The listing builds one solid part. Answer for the finished solid, in the listing's coordinates (mm). Face numbers are marked on the shaded views. A direction names the side the tool comes from. Give positions to 0.01 mm unless a question says otherwise; leave off trailing zeros. Order: outer loops, then holes, each group sorted by start corner. A loop starts at its lowest first (then second) coordinate and runs counter-clockwise, first axis right, second up. Notation, with made-up numbers: (65, 23) - (80, 23) arc R15 ccw to (80, 52) - close; hole circle Ø3 at (-11.5, -37). An arc over 180 degrees is marked (long way). Answer in a Markdown table with one row per item. Add a question column.
```python
from build123d import *

# Parameters (mm, degrees)
BOSS_EXTRUDE1_DEPTH = 220
CUT_EXTRUDE1_REACH  = 22
SKETCH3_R           = 3
CUT_EXTRUDE2_DEPTH  = 220


with BuildPart() as part:
    # Sketch1 → Boss-Extrude1 (new body)
    with BuildSketch(Plane.XY):
        Polygon((-157.703422053, 227.136882129), (-157.703422053, 225.136882129), (-177.703422053, 225.136882129), (-177.703422053, 250.136882129), (-157.703422053, 250.136882129), (-157.703422053, 248.136882129), (-175.703422053, 248.136882129), (-175.703422053, 227.136882129), align=None)
    extrude(amount=BOSS_EXTRUDE1_DEPTH)

    # Sketch2 → Cut-Extrude1 (cut, up to next)
    with BuildSketch(Plane.ZY.offset(177.703422053), mode=Mode.PRIVATE) as cut_extrude1_sk1:
        with BuildLine():
            Line((34.406705906, 248.069619472), (185.593294094, 248.069619472))
            ThreePointArc((185.593294094, 248.069619472), (196.026031437, 237.636882129), (185.593294094, 227.204144786))
            Line((185.593294094, 227.204144786), (34.406705906, 227.204144786))
            ThreePointArc((34.406705906, 227.204144786), (25.093294094, 237.636882129), (34.406705906, 248.069619472))
        make_face()
    cut_extrude1_tool1 = extrude(cut_extrude1_sk1.sketch, amount=-CUT_EXTRUDE1_REACH, mode=Mode.PRIVATE) & part.part
    add(cut_extrude1_tool1.solids().sort_by_distance((-177.703422, 237.636882, 110.543615))[0], mode=Mode.SUBTRACT)

    # Sketch3 → Cut-Extrude2 (cut)
    with BuildSketch(Plane(origin=(0, 250.136882129, 0), x_dir=(1, 0, 0), z_dir=(0, 1, 0))):
        with Locations((-170.703422053, -210)):
            Circle(SKETCH3_R)
        with Locations((-170.703422053, -10)):
            Circle(SKETCH3_R)
    extrude(amount=-CUT_EXTRUDE2_DEPTH, mode=Mode.SUBTRACT)


solid = part.part
```
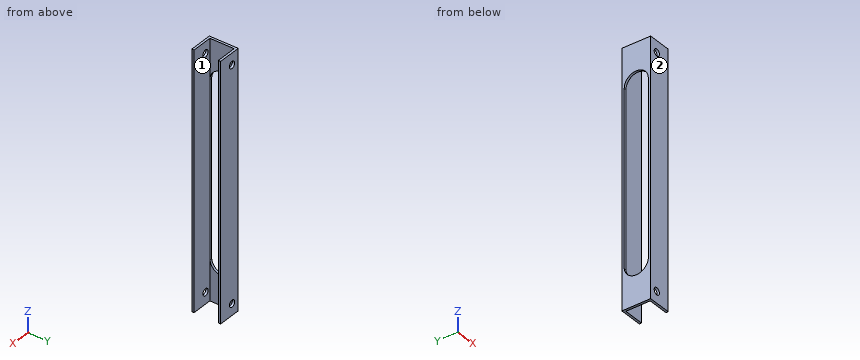
(1) For the marked faces 1 and 2, determine the directions among +Z, -Z, +X, -X, +Y, -Y from which every point of the face is accessible in a straight line to the end or side of a thin tool.
(2) Find section B-B, the plane z = 57.5. Write down the section's boundary in (x, y).
(3) Find section D-D, the plane z = 210. Write down the section's boundary in (x, y), plus the area to 3 significant figures.
(4) Find section C-C, the plane y = 241. Write down the section's boundary in (x, z), plus the area to 3 significant figures.
(5) Find section A-A, the plane x = -162.5. Write down the section's boundary in (y, z), plus the area to 3 significant figures.
(6) Straight lines are drawn through the part: line 1 (Y direction, x = -161, z = 69); line 2 (X direction, y = 249, z = 210); line 3 (Y direction, x = -175.75, z = 89). For each, find the intervals that lie inside material, in ascending order.
(7) Each of these flat-tipped pins is pushed along its axis until it touches: P1, Ø12, axis at x = -164, y = 234, coming from the +Z side; P2, Ø9.5, axis at x = -170.7, z = 210, coming from the -Y side. Where does it stop, or does it pass through?
Answer key:
| question | item | result |
|---|---|---|
| 1 | face 1 | +Z, -Z, +X |
| 1 | face 2 | +Z, -Z, +X, -X, -Y |
| 2 | outline | (-177.7, 225.14) - (-157.7, 225.14) - (-157.7, 227.14) - (-175.7, 227.14) - (-175.7, 227.2) - (-177.7, 227.2) - close; (-177.7, 248.07) - (-175.7, 248.07) - (-175.7, 248.14) - (-157.7, 248.14) - (-157.7, 250.14) - (-177.7, 250.14) - close |
| 3 | outline | (-177.7, 225.14) - (-173.7, 225.14) - (-173.7, 227.14) - (-175.7, 227.14) - (-175.7, 248.14) - (-173.7, 248.14) - (-173.7, 250.14) - (-177.7, 250.14) - close; (-167.7, 225.14) - (-157.7, 225.14) - (-157.7, 227.14) - (-167.7, 227.14) - close; (-167.7, 248.14) - (-157.7, 248.14) - (-157.7, 250.14) - (-167.7, 250.14) - close |
| 3 | area | 98.0 mm² |
| 4 | outline | (-177.7, 0) - (-175.7, 0) - (-175.7, 25.65) - (-177.7, 25.65) - close; (-177.7, 195.47) - (-175.7, 195.47) - (-175.7, 220) - (-177.7, 220) - close |
| 4 | area | 100 mm² |
| 5 | outline | (225.14, 0) - (227.14, 0) - (227.14, 220) - (225.14, 220) - close; (248.14, 0) - (250.14, 0) - (250.14, 220) - (248.14, 220) - close |
| 5 | area | 880 mm² |
| 6 | line 1 | 225.14 to 227.14, 248.14 to 250.14 |
| 6 | line 2 | -177.7 to -173.7, -167.7 to -157.7 |
| 6 | line 3 | 225.14 to 227.2, 248.07 to 250.14 |
| 7 | P1 | through |
| 7 | P2 | y = 225.14 |
